For this review, take the finished solid that the model builds, in its own axes (mm). A direction names the side the tool comes from. Coordinates: 2 decimals unless noted, no trailing zeros. Loops run counter-clockwise (first coordinate to the right, second up) from the corner with the lowest first, then second, coordinate; pieces in that order, holes last.
1. Machinability: for faces 1 (the face through (-11, 10, 2)), 2 (the face through (-24, 10, 2)), 3 (the face through (-21, 9, 5)), which of the approach directions +Z, -Z, +X, -X, +Y, -Y give a long, thin tool a straight path to every point of the face, cutting with its end or side? Answer none if there is none.
2. To check wall thickness, follow probe 1 along Z at (x, y) = (-8, 7.25); probe 2 along X at (y, z) = (8.25, 8.5); probe 3 along X at (y, z) = (7.5, 0.75). State the ranges of each line that lie inside material, in increasing order.
3. Clearance check with flat-ended pins moving along their axes: P1, Ø2.5, axis at x = -9.82, y = 8.31, coming from the -Z side; P2, Ø2.5, axis at x = -17.5, z = 7, coming from the -Y side; P3, Ø3, axis at x = -10.5, y = 9.5, coming from the -Z side; P4, Ø1, axis at y = 6, z = 2, coming from the +X side. State where each tip first meets the part, or that it passes through.
4. Take a section at B-B, the plane z = 8.5. State the section outline as (x, y) points, then the cut area to 3 significant figures.
5. Take a section at D-D, the plane y = 10.5. State the section outline as (x, z) points.
6. Take a section at A-A, the plane x = -8. State the section outline as (y, z) points.
7. Mouldability with a two-part tool opening along X and no side actions: class faces 4 (the face through (-17, 9.314, 5)), 5 (the face through (-13, 9, 0)), 6 (the face through (-12.78, 10.19, 4.96)), 7 (the face through (-21.896, 10.23, 0.986)) as pulls with the +X half, pulls with the -X half, needs draft (parallel to the pull), parting line crosses it, or undercut.
8. Take a section at C-C, the plane x = -11. State the section outline as (y, z) points, then the cut area to 3 significant figures.
```python
from build123d import *

# Parameters (mm, degrees)
ESTRUSIONE_ESTRUSIONE1_DEPTH = 10
SCHIZZO5_R                   = 1.499999999999997
SCHIZZO5_R_2                 = 1.5000000000000009
TAGLIO_ESTRUSIONE1_DEPTH     = 10
SCHIZZO6_R                   = 3.4999999999999996
TAGLIO_ESTRUSIONE2_DEPTH     = 2
TAGLIO_ESTRUSIONE3_START     = -8
SCHIZZO6_2_R                 = 3.4999999999999996
TAGLIO_ESTRUSIONE3_DEPTH     = 12
TAGLIO_ESTRUSIONE4_START     = -2
SCHIZZO7_R                   = 3.4999999999999996
TAGLIO_ESTRUSIONE4_DEPTH     = 6
RACCORDO1_R                  = 2
RACCORDO2_R                  = 2


with BuildPart() as part:
    # Schizzo1 → Estrusione-Estrusione1 (new body)
    with BuildSketch(Plane.XY):
        with BuildLine():
            Line((-24.824967096652905, 11.313668704827196), (-9.824967096652905, 11.313668704827196))
            ThreePointArc((-9.824967096652905, 11.313668704827196), (-8.092916289084027, 5.864178962044019), (-12.653394221399095, 9.313668704827194))
            Line((-12.653394221399095, 9.313668704827194), (-21.996539971906714, 9.313668704827194))
            ThreePointArc((-21.996539971906714, 9.313668704827194), (-26.557017904221784, 5.864178962044019), (-24.824967096652905, 11.313668704827196))
        make_face()
    extrude(amount=ESTRUSIONE_ESTRUSIONE1_DEPTH)

    # Schizzo5 → Taglio-Estrusione1 (cut)
    with BuildSketch(Plane(origin=(0, 0, 0), x_dir=(-1, 0, 0), z_dir=(0, 0, -1))):
        with Locations((9.824967096652905, 8.313668704827196)):
            Circle(SCHIZZO5_R)
        with Locations((24.824967096652905, 8.313668704827196)):
            Circle(SCHIZZO5_R_2)
    extrude(amount=-TAGLIO_ESTRUSIONE1_DEPTH, mode=Mode.SUBTRACT)

    # Schizzo6 → Taglio-Estrusione2 (cut)
    with BuildSketch(Plane(origin=(0, 0, 0), x_dir=(-1, 0, 0), z_dir=(0, 0, -1))):
        with Locations((24.824967096652905, 8.313668704827196)):
            Circle(SCHIZZO6_R)
    extrude(amount=-TAGLIO_ESTRUSIONE2_DEPTH, mode=Mode.SUBTRACT)

    # Schizzo6<2> → Taglio-Estrusione3 (cut)
    with BuildSketch(Plane(origin=(0, 0, 0), x_dir=(-1, 0, 0), z_dir=(0, 0, -1)).offset(TAGLIO_ESTRUSIONE3_START)):
        with Locations((24.824967096652905, 8.313668704827196)):
            Circle(SCHIZZO6_2_R)
    extrude(amount=-TAGLIO_ESTRUSIONE3_DEPTH, mode=Mode.SUBTRACT)

    # Schizzo7 → Taglio-Estrusione4 (cut)
    with BuildSketch(Plane(origin=(0, 0, 0), x_dir=(-1, 0, 0), z_dir=(0, 0, -1)).offset(TAGLIO_ESTRUSIONE4_START)):
        with Locations((9.824967096652905, 8.313668704827196)):
            Circle(SCHIZZO7_R)
    extrude(amount=-TAGLIO_ESTRUSIONE4_DEPTH, mode=Mode.SUBTRACT)

    # Raccordo1
    raccordo1_edges = [part.edges().sort_by_distance(p)[0] for p in [
        (-21.996539971906714, 9.313668704827194, 5),
    ]]
    fillet(raccordo1_edges, radius=RACCORDO1_R)

    # Raccordo2
    raccordo2_edges = [part.edges().sort_by_distance(p)[0] for p in [
        (-12.653394221399093, 9.313668704827194, 1),
    ]]
    fillet(raccordo2_edges, radius=RACCORDO2_R - 0.0001)  # a hair under: the kernel refuses the full size


solid = part.part
```
Results list:
1. face 1: +X, -Y
1. face 2: -Z, -X, -Y
1. face 3: +Z, -Z, -Y
2. probe 1: z = 0 to 2, 8 to 10
2. probe 2: x = -12.96 to -11.32, -8.33 to -6.83
2. probe 3: x = -12.71 to -11.09, -8.56 to -6.94
3. P1: passes through
3. P2: stops at y = 9.31
3. P3: stops at z = 0
3. P4: stops at x = -7.44
4. outline: (-23.02, 11.31) arc R3.5 cw to (-21.35, 8.72) arc R2 cw to (-19.93, 9.31) - (-14.72, 9.31) arc R2 cw to (-12.76, 7.71) arc R3 ccw (long way) to (-9.82, 11.31) - close; hole circle Ø3 at (-9.82, 8.31)
4. area: 42.6 mm2
5. outline: (-26.88, 2) - (-22.09, 2) - (-22.09, 0) - (-7.77, 0) - (-7.77, 2) - (-12.56, 2) - (-12.56, 8) - (-7.77, 8) - (-7.77, 10) - (-22.09, 10) - (-22.09, 8) - (-26.88, 8) - close
6. outline: (5.93, 0) - (10.69, 0) - (10.69, 2) - (5.93, 2) - close; (5.93, 8) - (10.69, 8) - (10.69, 10) - (5.93, 10) - close
7. face 4: undercut
7. face 5: needs draft
7. face 6: pulls with the +X half
7. face 7: pulls with the -X half
8. outline: (5.55, 0) - (7.38, 0) - (7.38, 2) - (5.55, 2) - close; (5.55, 8) - (7.38, 8) - (7.38, 10) - (5.55, 10) - close; (9.25, 0) - (11.31, 0) - (11.31, 2) - (9.25, 2) - close; (9.25, 8) - (11.31, 8) - (11.31, 10) - (9.25, 10) - close
8. area: 15.6 mm2
